Model file for the job. Use its own axes, mm. Face numbers are marked on the shaded views. Give positions to 0.01 mm unless a question says otherwise; leave off trailing zeros. Order: outer loops, then holes, each group sorted by start corner. A loop starts at its lowest first (then second) coordinate and runs counter-clockwise, first axis right, second up. Notation, with made-up numbers: (35.5, 50.5) - (90.5, 50.5) arc R37 cw to (90.5, 86.5) - close; hole circle Ø9 at (12.5, -37.75). An arc over 180 degrees is marked (long way). Use CSV: the item, a comma, the result in double quotes. Start each with the question number.
(1) Band-saw the part on A-A, the plane x = 0. Give the cut face in (y, z).
(2) Pull direction X, two halves, no side cores. Call the marked faces 1 and 2: +X half, -X half, draft (parallel to the pull), parting line (faces both ways), or undercut.
(3) Probe L1, parallel to X at y = 160, z = 0; L2, parallel to Z at x = -1, y = 64; L3, parallel to X at y = 150.5, z = -1. List the from-to ranges inside material, lowest first.
(4) Drop flat-ended pins along their axis: pin 1 Ø1 at (x, y) = (9, 111) entering from +Z; pin 2 Ø8 at (x, y) = (13, 104.5) entering from +Z; pin 3 Ø1.5 at (y, z) = (132, 19.5) entering from +X. Give the stop position or say it passes through.
(5) Band-saw the part on C-C, the plane y = 132.5. Give the cut face in (x, z), then the cut area to 3 significant figures.
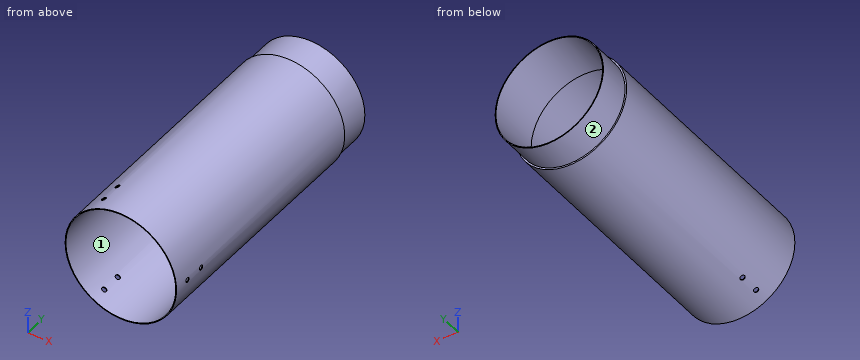
Autodesk Inventor part; units mm, degrees
ref_plane "Work Plane2" through (35, 0, 0) normal (1, 0, 0) x (0, 1, 0)
ref_plane "Work Plane4" through (34, 0, 0) normal (1, 0, 0) x (0, 1, 0)
ref_plane "XZ Plane" through (0, 0, 0) normal (0, 1, 0) x (-1, 0, 0)
sketch "Sketch1" plane through (0, 0, 0) normal (0, 1, 0) x (-1, 0, 0)
  circle A0 centre (0, 0) radius 35
  circle A1 centre (0, 0) radius 34.5
  dimension "d0" = 70
  dimension "d1" = 69
extrude "Extrusion1" add sketch "Sketch1" along normal blind 155
ref_plane "Work Plane2" through (35, 0, 0) normal (1, 0, 0) x (0, 1, 0)
sketch "Sketch4" plane through (35, 0, 0) normal (1, 0, 0) x (0, 1, 0)
  line L0 (155, -35) -> (155, 35)
  point P0 (0, 0)
  point P1 (10, 0)
  dimension "d48" = 10
hole "Hole2" at (35, 10, 0) direction (-1, 0, 0) diameter 3 depth 8 tip angle 118
sketch "Sketch5" plane through (0, 155, 0) normal (0, 1, 0) x (1, 0, 0)
  circle A0 centre (0, 0) radius 34
  circle A1 centre (0, 0) radius 33.5
  dimension "d44" = 68
  dimension "d45" = 67
extrude "Extrusion3" add sketch "Sketch5" along normal blind 20
sketch "Sketch6" plane through (0, 155, 0) normal (0, -1, 0) x (1, 0, 0)
  circle A0 centre (0, 0) radius 33.5
  circle A1 centre (0, 0) radius 34.5
  circle A2 centre (0, 0) radius 35
extrude "Extrusion4" add sketch "Sketch6" along normal blind 12.5 contours A1
ref_plane "Work Plane4" through (34, 0, 0) normal (1, 0, 0) x (0, 1, 0)
pattern_circular "Circular Pattern2" count 3 over 360 about axis through (0, 0, 0) along (0, 1, 0) of "Hole2"
sketch "Sketch10" plane through (35, 0, 0) normal (1, 0, 0) x (0, 1, 0)
  point P0 (0, 0)
  point P1 (22.5, 0)
  dimension "d82" = 22.5
hole "Hole6" at (35, 22.5, 0) direction (-1, 0, 0) diameter 3 depth 8 tip angle 118
pattern_circular "Circular Pattern3" count 3 over 360 about axis through (0, 0, 0) along (0, 1, 0) of "Hole6"
properties part number "Engine skin" material "Plastic, Opaque White"
Answer block:
1,outline,"(0, -35) - (155, -35) - (155, -34) - (175, -34) - (175, -33.5) - (142.5, -33.5) - (142.5, -34.5) - (0, -34.5) - close; (0, 34.5) - (142.5, 34.5) - (142.5, 33.5) - (175, 33.5) - (175, 34) - (155, 34) - (155, 35) - (0, 35) - close"
2,face 1,"undercut"
2,face 2,"parting line"
3,L1,"x = -34 to -33.5, 33.5 to 34"
3,L2,"z = -34.99 to -34.49, 34.49 to 34.99"
3,L3,"x = -34.99 to -33.49, 33.49 to 34.99"
4,pin 1,"stops at z = 33.95"
4,pin 2,"stops at z = 33.82"
4,pin 3,"stops at x = 29.55"
5,outline,"circle Ø70 at (0, 0); hole circle Ø69 at (0, 0)"
5,area,"109 mm2"
